Geometry check sheet. Reference: the model listing, model coordinates, mm. A direction names the side the tool comes from. Round coordinates to 2 decimals unless told otherwise and drop trailing zeros. Order: outer loops, then holes, each group sorted by start corner. A loop starts at its lowest first (then second) coordinate and runs counter-clockwise, first axis right, second up.
(1) Sectioned sample at C-C (x = -58.5). Record the boundary of the cut face in (y, z), plus the area to 3 significant figures.
(2) Set-up check for faces 1 (the face through (20, 20, -25)), 2 (the face through (49, 20, -13)), 3 (the face through (0, 7, -49)), 4 (the face through (23, 20, -18)): record each of +Z, -Z, +X, -X, +Y, -Y from which the full face is reachable in a straight line by a thin tool's end or side.
(3) Sectioned sample at A-A (z = 1). Record the boundary of the cut face in (x, y).
(4) Release check for a two-part mould opening along Y. For faces 5 (the face through (0, 2, -5)), 6 (the face through (-14, 20, -70)), 7 (the face through (0, 40, -5)), 8 (the face through (0, 0, -5)) record: +Y half, -Y half, draft (parallel to the pull), parting line (faces both ways), or undercut.
(5) Sectioned sample at D-D (x = -10). Record the boundary of the cut face in (y, z), plus the area to 3 significant figures.
(6) Sectioned sample at B-B (z = -63). Record the boundary of the cut face in (x, y), plus the area to 3 significant figures.
(7) Material ranges on line 1 along X through (y, z) = (9, -61); line 2 along X through (y, z) = (27, 14.5), recorded low to high.
(8) Go/stop test with flat-tipped pins: pin 1 (10 mm diameter, centred on x = -44.5, y = 32, fed in from -Z); pin 2 (1.5 mm diameter, centred on x = 28, y = 18, fed in from -Z); pin 3 (8 mm diameter, centred on y = 16, z = -52.5, fed in from -X); pin 4 (23 mm diameter, centred on x = 10, z = 1, fed in from -Y). Record where each tip stops, or that it passes through.
from build123d import *

# Parameters (mm, degrees)
CROQUIS1_W     = 40
CROQUIS1_H     = 50
CROQUIS1_H_2   = 40
CROQUIS1_W_2   = 50
EXTRUIR1_DEPTH = 40
CROQUIS2_W     = 40
CROQUIS2_H     = 40
CROQUIS2_W_2   = 30
CROQUIS2_H_2   = 30
EXTRUIR2_DEPTH = 40
CROQUIS3_W     = 40
CROQUIS3_H     = 40
CROQUIS3_W_2   = 30
CROQUIS3_H_2   = 30
EXTRUIR3_DEPTH = 40
CROQUIS5_W     = 40
CROQUIS5_H     = 40
CROQUIS5_W_2   = 30
CROQUIS5_H_2   = 30
EXTRUIR4_DEPTH = 40
VACIADO1_T     = -2


with BuildPart() as part:
    # Croquis1 → Extruir1 (new body)
    with BuildSketch(Plane(origin=(0, 0, 0), x_dir=(1, 0, 0), z_dir=(0, 1, 0))):
        with Locations((0, 45)):
            Rectangle(CROQUIS1_W, CROQUIS1_H)
        Rectangle(CROQUIS1_W, CROQUIS1_H_2)
        with Locations((45, 0)):
            Rectangle(CROQUIS1_W_2, CROQUIS1_H_2)
        with Locations((-45, 0)):
            Rectangle(CROQUIS1_W_2, CROQUIS1_H_2)
    extrude(amount=EXTRUIR1_DEPTH)

    # Croquis2 → Extruir2 (cut)
    with BuildSketch(Plane(origin=(70, 0, 0), x_dir=(0, 0, -1), z_dir=(1, 0, 0))):
        with Locations((0, 20)):
            Rectangle(CROQUIS2_W, CROQUIS2_H)
        with Locations((0, 20)):
            Rectangle(CROQUIS2_W_2, CROQUIS2_H_2, mode=Mode.SUBTRACT)
    extrude(amount=-EXTRUIR2_DEPTH, mode=Mode.SUBTRACT)

    # Croquis3 → Extruir3 (cut)
    with BuildSketch(Plane(origin=(0, 0, -70), x_dir=(-1, 0, 0), z_dir=(0, 0, -1))):
        with Locations((0, 20)):
            Rectangle(CROQUIS3_W, CROQUIS3_H)
        with Locations((0, 20)):
            Rectangle(CROQUIS3_W_2, CROQUIS3_H_2, mode=Mode.SUBTRACT)
    extrude(amount=-EXTRUIR3_DEPTH, mode=Mode.SUBTRACT)

    # Croquis5 → Extruir4 (cut)
    with BuildSketch(Plane.ZY.offset(70)):
        with Locations((0, 20)):
            Rectangle(CROQUIS5_W, CROQUIS5_H)
        with Locations((0, 20)):
            Rectangle(CROQUIS5_W_2, CROQUIS5_H_2, mode=Mode.SUBTRACT)
    extrude(amount=-EXTRUIR4_DEPTH, mode=Mode.SUBTRACT)

    # Vaciado1
    vaciado1_openings = [part.faces().sort_by_distance(p)[0] for p in [
        (70, 20, 0),
        (0, 20, -70),
        (-70, 20, 0),
    ]]
    offset(amount=VACIADO1_T, openings=vaciado1_openings, kind=Kind.INTERSECTION)


solid = part.part
Answer below:
1. outline: (5, -15) - (35, -15) - (35, 15) - (5, 15) - close; hole (7, -13) - (33, -13) - (33, 13) - (7, 13) - close
1. area: 224 mm2
2. face 1: -Z, +X, +Y, -Y
2. face 2: +X, -X
2. face 3: -Z
2. face 4: none
3. outline: (-70, 5) - (-30, 5) - (-30, 0) - (30, 0) - (30, 5) - (70, 5) - (70, 7) - (28, 7) - (28, 2) - (-28, 2) - (-28, 7) - (-70, 7) - close; (-70, 33) - (-28, 33) - (-28, 38) - (28, 38) - (28, 33) - (70, 33) - (70, 35) - (30, 35) - (30, 40) - (-30, 40) - (-30, 35) - (-70, 35) - close
4. face 5: undercut
4. face 6: draft
4. face 7: +Y half
4. face 8: -Y half
5. outline: (0, -30) - (5, -30) - (5, -70) - (7, -70) - (7, -28) - (2, -28) - (2, 18) - (38, 18) - (38, -28) - (33, -28) - (33, -70) - (35, -70) - (35, -30) - (40, -30) - (40, 20) - (0, 20) - close
5. area: 452 mm2
6. outline: (-15, 5) - (15, 5) - (15, 35) - (-15, 35) - close; hole (-13, 7) - (13, 7) - (13, 33) - (-13, 33) - close
6. area: 224 mm2
7. line 1: x = -15 to -13, 13 to 15
7. line 2: x = -70 to -28, 28 to 70
8. pin 1: stops at z = -15
8. pin 2: stops at z = -20
8. pin 3: stops at x = -15
8. pin 4: stops at y = 0
